```python
from build123d import *

# Parameters (mm, degrees)
SKETCH1_W           = 64.5
SKETCH1_H           = 45.5
SKETCH1_W_2         = 8.5
SKETCH1_H_2         = 8.5
BOSS_EXTRUDE1_DEPTH = 2
SKETCH2_W           = 64.5
SKETCH2_H           = 45.5
SKETCH2_W_2         = 28
SKETCH2_H_2         = 41.5
BOSS_EXTRUDE2_DEPTH = 14
CUT_EXTRUDE1_REACH  = 80.565
SKETCH3_R           = 14
SKETCH4_W           = 1.5
SKETCH4_H           = 38.5
BOSS_EXTRUDE3_DEPTH = 5
SKETCH5_W           = 15.24
SKETCH5_H           = 2
CUT_EXTRUDE2_DEPTH  = 7.62


with BuildPart() as part:
    # Sketch1 → Boss-Extrude1 (new body)
    with BuildSketch(Plane(origin=(0, 0, 0), x_dir=(0, 0, -1), z_dir=(1, 0, 0))):
        with Locations((30.25, 20.75)):
            Rectangle(SKETCH1_W, SKETCH1_H)
        with Locations((46.5590026, 29.024)):
            Rectangle(SKETCH1_W_2, SKETCH1_H_2, mode=Mode.SUBTRACT)
    extrude(amount=BOSS_EXTRUDE1_DEPTH)

    # Sketch2 → Boss-Extrude2 (add)
    with BuildSketch(Plane.ZY):
        with Locations((-30.25, 20.75)):
            Rectangle(SKETCH2_W, SKETCH2_H)
        with Locations((-46.5, 20.75)):
            Rectangle(SKETCH2_W_2, SKETCH2_H_2, mode=Mode.SUBTRACT)
        with Locations((-14, 20.75)):
            Rectangle(SKETCH2_W_2, SKETCH2_H_2, mode=Mode.SUBTRACT)
    extrude(amount=BOSS_EXTRUDE2_DEPTH)

    # Sketch3 → Cut-Extrude1 (cut, up to next)
    with BuildSketch(Plane(origin=(0, 43.5, 0), x_dir=(1, 0, 0), z_dir=(0, 1, 0)), mode=Mode.PRIVATE) as cut_extrude1_sk1:
        with Locations((-14, 14)):
            Circle(SKETCH3_R)
    cut_extrude1_tool1 = extrude(cut_extrude1_sk1.sketch, amount=-CUT_EXTRUDE1_REACH, mode=Mode.PRIVATE) & part.part
    add(cut_extrude1_tool1.solids().sort_by_distance((-14, 43.5, -14))[0], mode=Mode.SUBTRACT)

    # Sketch4 → Boss-Extrude3 (add)
    with BuildSketch(Plane.ZY.offset(14)):
        with Locations((-30.25, 20.75)):
            Rectangle(SKETCH4_W, SKETCH4_H)
    extrude(amount=BOSS_EXTRUDE3_DEPTH)

    # Sketch5 → Cut-Extrude2 (cut)
    with BuildSketch(Plane.ZY.offset(14)):
        with Locations((-47.26, -1)):
            Rectangle(SKETCH5_W, SKETCH5_H)
    extrude(amount=-CUT_EXTRUDE2_DEPTH, mode=Mode.SUBTRACT)


solid = part.part
```
Check sheet for the modelled part. Datum: model origin and axes. Units: mm. A direction names the side the tool comes from. Give positions to 0.01 mm unless a question says otherwise; leave off trailing zeros. Write each loop counter-clockwise with the first axis right and the second up, starting at its lowest first coordinate (ties: lowest second). Pieces come first, ordered by that corner, then holes. Notation, with made-up numbers: (50.25, 8.25) - (109.25, 8.25) arc R17 ccw to (109.25, 32.25) - close; hole circle Ø3 at (16.5, -14.75). An arc over 180 degrees is marked (long way). Answer as a JSON object with one key per item and string values. Group by question number.
1) Depth check by flat-ended pin: P1, Ø8.5, axis at y = 13.5, z = -45, coming from the -X side; P2, Ø1.5, axis at x = -16.5, y = 27, coming from the -Z side; P3, Ø1.5, axis at x = -1.5, z = -14.5, coming from the +Y side. Enter the tip coordinate at first touch or a pass-through.
2) Sectioned sample at C-C (x = -16.25). Record the cut outline in (y, z).
3) Release check for a two-part mould opening along Z. For faces 1 (the face through (-16, 20, -31)), 2 (the face through (-3, 41.5, -3)), 3 (the face through (-16, 40, -30)) record: pulls with the +Z half, pulls with the -Z half, needs draft (parallel to the pull), parting line crosses it, or undercut.
4) Thickness scan on probe 1 along Z at (x, y) = (-4, 18); probe 2 along Y at (x, z) = (-3, -23); probe 3 along X at (y, z) = (31.5, -27.5). Record the ranges inside material, lowest first. Write a range as from..to.
5) Access from +Z, -Z, +X, -X, +Y, -Y to the whole of each face (thin tool, end or side, straight path). Record for faces 4 (the face through (-3, 41.5, -25)), 5 (the face through (-16, 1.5, -30)), 6 (the face through (1, 33.274, -46)), 7 (the face through (-10, -1, -39.64)).
6) Sectioned sample at A-A (y = 12). Record the cut outline in (x, z).
7) Sectioned sample at D-D (z = -16). Record the cut outline in (x, y), then the cut area to 3 significant figures.
8) Sectioned sample at B-B (z = -3). Record the cut outline in (x, y), then the cut area to 3 significant figures.
Geometry results:
{
 "1": {"P1": "stops at x = 0", "P2": "stops at z = -31", "P3": "stops at y = 0"},
 "2": {"outline": "(1.5, -31) - (40, -31) - (40, -29.5) - (1.5, -29.5) - close"},
 "3": {"face 1": "pulls with the -Z half", "face 2": "undercut", "face 3": "needs draft"},
 "4": {"probe 1": "z = -62.5..-60.5, -32.5..-28, 0..2", "probe 2": "y = -2..0, 41.5..43.5", "probe 3": "x = 0..2"},
 "5": {"face 4": "-X", "face 5": "+Z, -Z, -X, -Y", "face 6": "+X, -X", "face 7": "-X, -Y"},
 "6": {"outline": "(-19, -31) - (-14, -31) - (-14, -32.5) - (0, -32.5) - (0, -60.5) - (-14, -60.5) - (-14, -62.5) - (2, -62.5) - (2, 2) - (-14, 2) - (-14, 0) - (0, 0) - (0, -28) - (-14, -28) - (-14, -29.5) - (-19, -29.5) - close"},
 "7": {"outline": "(-14, -2) - (2, -2) - (2, 43.5) - (-0.14, 43.5) - (-0.14, 41.5) - (0, 41.5) - (0, 0) - (-14, 0) - close", "area": "119 mm^2"},
 "8": {"outline": "(-14, -2) - (2, -2) - (2, 43.5) - (-5.34, 43.5) - (-5.34, 41.5) - (0, 41.5) - (0, 0) - (-14, 0) - close", "area": "130 mm^2"}
}
